from build123d import *

# Parameters (mm, degrees)
F0_W      = 101.6
F0_H      = 58.316330242
F2_DEPTH  = 25.4
F1_W      = 50.8
F1_H      = 12.7
F3_DEPTH  = 50.8
F5_R      = 12.7
F4_R      = 10.16
F6_DEPTH  = 6.35
F8_R      = 1.27
F10_DEPTH = 12.7
F12_DEPTH = 12.701
F13_R     = 20.32
F14_R     = 5.715
F15_DEPTH = 19.051


with BuildPart() as f2:
    # F0 (on Front) → F2 (new body)
    with BuildSketch(Plane.XZ):
        with Locations((0, 29.158165121)):
            Rectangle(F0_W, F0_H)
    extrude(amount=F2_DEPTH)

    # F1 (on Front) → F3 (join)
    with BuildSketch(Plane.XZ):
        with Locations((-50.8, 6.35)):
            Rectangle(F1_W, F1_H)
        with Locations((50.8, 6.35)):
            Rectangle(F1_W, F1_H)
    extrude(amount=F3_DEPTH)

    # F5
    f5_edges = [f2.edges().sort_by_distance(p)[0] for p in [
        (-76.2, -50.8, 6.35),
        (-25.4, -50.8, 6.35),
        (25.4, -50.8, 6.35),
        (76.2, -50.8, 6.35),
    ]]
    fillet(f5_edges, radius=F5_R)

    # F4 (on face) → F6 (join)
    with BuildSketch(Plane.XY.offset(12.7)):
        with Locations((-50.8, -38.1)):
            Circle(F4_R)
    extrude(amount=F6_DEPTH)

    # F7: F2 across plane


with BuildPart() as f2_1:
    add(f2.part)
    add(f2.part.mirror(Plane.YZ))

    # F8
    f8_edges = [f2_1.edges().sort_by_distance(p)[0] for p in [
        (-60.96, -38.1, 19.05),
        (60.96, -38.1, 19.05),
    ]]
    fillet(f8_edges, radius=F8_R)

    # F9 (on face) → F10 (cut)
    with BuildSketch(Plane.XZ.offset(25.4)):
        with BuildLine():
            ThreePointArc((-38.1, 58.316330242), (0, 20.216330242), (38.1, 58.316330242))
            Line((38.1, 58.316330242), (-38.1, 58.316330242))
        make_face()
    extrude(amount=-F10_DEPTH, mode=Mode.SUBTRACT)

    # F11 (on face) → F12 (cut, through all)
    with BuildSketch(Plane.XZ.offset(12.7)):
        with BuildLine():
            ThreePointArc((-25.4, 58.316330242), (0, 32.916330242), (25.4, 58.316330242))
            Line((25.4, 58.316330242), (-25.4, 58.316330242))
        make_face()
    extrude(amount=-F12_DEPTH, mode=Mode.SUBTRACT)

    # F13
    f13_edges = [f2_1.edges().sort_by_distance(p)[0] for p in [
        (50.8, -12.7, 12.7),
        (-50.8, -12.7, 12.7),
    ]]
    fillet(f13_edges, radius=F13_R)

    # F14 (on face) → F15 (cut, through all)
    with BuildSketch(Plane.XY.offset(19.05)):
        with Locations((-50.8, -38.1)):
            Circle(F14_R)
        with Locations((50.8, -38.1)):
            Circle(F14_R)
    extrude(amount=-F15_DEPTH, mode=Mode.SUBTRACT)


solid = f2_1.part
Geometry: final body of the model. Coordinates: model frame, mm. A direction names the side the tool comes from. Give positions to 0.01 mm unless a question says otherwise; leave off trailing zeros. Order: outer loops, then holes, each group sorted by start corner. A loop starts at its lowest first (then second) coordinate and runs counter-clockwise, first axis right, second up. Notation, with made-up numbers: (77.25, -18) -> (128.25, -18) arc R7 ccw to (128.25, -11) -> close; hole circle Ø6 at (4, 2). An arc over 180 degrees is marked (long way). Put each result on its own line as item: value.
Q1. Section D-D, the plane z = 24. Return loops of the section in (x, y).
Here are the results:
outline: (-52.91, -25.4) -> (-16.55, -25.4) -> (-16.55, -12.7) -> (16.55, -12.7) -> (16.55, -25.4) -> (52.91, -25.4) -> (52.91, 0) -> (-52.91, 0) -> close
Q2. Draft query along X for faces 5 (the face through (72.38, -47.18, 6.44)), 6 (the face through (-51, -50.8, 6)), 7 (the face through (-48.16, -43.17, 9.66)). Return one class per face: released by +X, released by -X, zero draft, split by the parting line, or undercut.
Here are the results:
face 5: released by +X
face 6: zero draft
face 7: undercut
Q3. Material intervals for L1, parallel to X at y = -38, z = 8; L2, parallel to X at y = -29.5, z = 4; L3, parallel to Y at x = 34.5, z = 42.5, sorted ascending.
Here are the results:
L1: x = -76.2 to -56.51, -45.09 to -25.4, 25.4 to 45.09, 56.51 to 76.2
L2: x = -76.2 to -25.4, 25.4 to 76.2
L3: y = -12.7 to 0
Q4. Section B-B, the plane z = 53.5. Return loops of the section in (x, y), then the cut area to 3 significant figures.
Here are the results:
outline: (-50.8, -25.4) -> (-37.79, -25.4) -> (-37.79, -12.7) -> (-24.94, -12.7) -> (-24.94, 0) -> (-50.8, 0) -> close; (24.94, -12.7) -> (37.79, -12.7) -> (37.79, -25.4) -> (50.8, -25.4) -> (50.8, 0) -> (24.94, 0) -> close
area: 987 mm^2
Q5. Section C-C, the plane x = 0. Return loops of the section in (y, z), then the cut area to 3 significant figures.
Here are the results:
outline: (-25.4, 0) -> (0, 0) -> (0, 32.92) -> (-12.7, 32.92) -> (-12.7, 20.22) -> (-25.4, 20.22) -> close
area: 675 mm^2
Q6. Pin query (flat end, axial travel): pin 1 (6 mm diameter, centred on x = 45.5, y = -42.5, fed in from +Z); pin 2 (20 mm diameter, centred on y = -18.5, z = 42, fed in from +X); pin 3 (2 mm diameter, centred on y = -18.5, z = 19, fed in from +X). Return the tip coordinate at first contact, or that it passes through.
Here are the results:
pin 1: stops at z = 19.05
pin 2: stops at x = 50.83
pin 3: stops at x = 57.43
Q7. Section A-A, the plane y = -4. Return loops of the section in (x, z).
Here are the results:
outline: (-76.2, 0) -> (76.2, 0) -> (76.2, 12.7) -> (71.12, 12.7) arc R20.32 cw to (50.8, 33.02) -> (50.8, 58.32) -> (25.4, 58.32) arc R25.4 cw to (-25.4, 58.32) -> (-50.8, 58.32) -> (-50.8, 33.02) arc R20.32 cw to (-71.12, 12.7) -> (-76.2, 12.7) -> close
Q8. Reachability of faces 1 (the face through (58.863, -44.282, 15.204)), 2 (the face through (29.02, -46.98, 6.44)), 3 (the face through (-0.838, -19.139, 20.226)), 4 (the face through (-50.8, -13, 45)) from +Z, -Z, +X, -X, +Y, -Y: full face, straight path, thin tool, end or side. Return the list, or none.
Here are the results:
face 1: +Z
face 2: +Z, -Z, -Y
face 3: +Z, -Y
face 4: +Z, -X, +Y, -Y
